Autodesk Inventor part; units mm, degrees
ref_plane "YZ Plane" through (0, 0, 0) normal (1, 0, 0) x (0, 1, 0)
ref_plane "XZ Plane" through (0, 0, 0) normal (0, 1, 0) x (-1, 0, 0)
ref_plane "XY Plane" through (0, 0, 0) normal (0, 0, 1) x (1, 0, 0)
sketch "Sketch1" plane through (0, 0, 0) normal (0, 1, 0) x (-1, 0, 0)
  line L0 (0, 0) -> (20, 0)
  line L1 (20, 0) -> (20, -20)
  line L2 (20, -20) -> (0, -20)
  line L3 (0, -20) -> (0, 0)
  dimension "d0" = 20
  dimension "d1" = 20
extrude "Extrusion1" add sketch "Sketch1" along normal blind 2
sketch "Sketch2" plane through (0, 2, 0) normal (0, 1, 0) x (1, 0, 0)
  line L0 (0, 20) -> (-20, 20)
  line L1 (-20, 20) -> (-20, 0)
  line L2 (-20, 0) -> (0, 0)
  line L3 (0, 0) -> (0, 20)
  line L4 (-18, 2) -> (-18, 18)
  line L5 (-18, 18) -> (-2, 18)
  line L6 (-2, 18) -> (-2, 2)
  line L7 (-2, 2) -> (-18, 2)
  line L8 (-16.75, 16.75) -> (-16.75, 3.25)
  line L9 (-16.75, 3.25) -> (-3.25, 3.25)
  line L10 (-3.25, 3.25) -> (-3.25, 16.75)
  line L11 (-3.25, 16.75) -> (-16.75, 16.75)
  dimension "d4" = 2
  dimension "d5" = 1.25
extrude "Extrusion2" add sketch "Sketch2" along normal blind 2 contours L4 L5 L6 L7
extrude "Extrusion3" cut sketch "Sketch2" against normal blind 10 contours L11 L10 L9 L8
sketch "Sketch3" plane through (0, 0, 0) normal (0, -1, 0) x (1, 0, 0)
  line L0 (-3.25, -3.25) -> (-3.25, -16.75)
  line L1 (-3.25, -16.75) -> (-16.75, -16.75)
  line L2 (-16.75, -16.75) -> (-16.75, -3.25)
  line L3 (-16.75, -3.25) -> (-3.25, -3.25)
  line L4 (0, -20) -> (-20, -20)
  line L5 (0, 0) -> (0, -20)
  line L6 (-20, 0) -> (0, 0)
  line L7 (-20, -20) -> (-20, 0)
  line L8 (-6, -6) -> (-6, -14)
  line L9 (-6, -14) -> (-14, -14)
  line L10 (-14, -14) -> (-14, -6)
  line L11 (-14, -6) -> (-6, -6)
extrude "Extrusion4" add sketch "Sketch3" against normal up to surface (2 mm away) contours L0 L1 L2 L3
extrude "Extrusion5" add sketch "Sketch3" against normal blind 11.5 contours L8 L9 L10 L11
properties part number "latticeChamberCapv4"
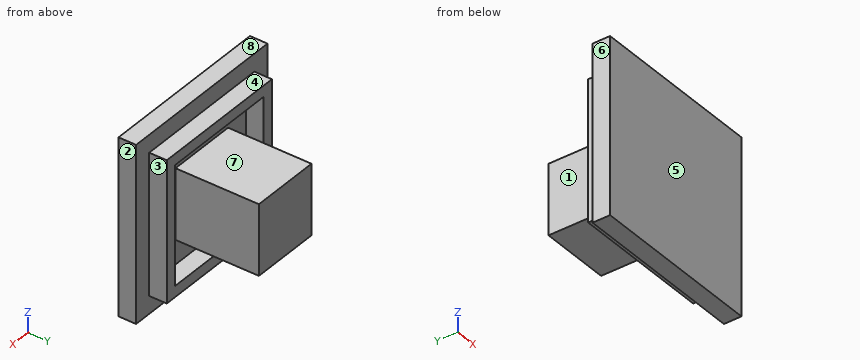
The listing builds one solid part. Answer for the finished solid, in the listing's coordinates (mm). Face numbers are marked on the shaded views. A direction names the side the tool comes from. Coordinates: 2 decimals unless noted, no trailing zeros. Write each loop counter-clockwise with the first axis right and the second up, starting at its lowest first coordinate (ties: lowest second). Pieces come first, ordered by that corner, then holes. Notation, with made-up numbers: (53, 69.5) - (90, 69.5) arc R23 ccw to (90, 98.5) - close; hole circle Ø1 at (29.5, -17.75). An arc over 180 degrees is marked (long way). One line per item, written item: value.
1) A tool of negligible diameter and unlimited length cuts with its end or side. For the marked faces 1, 2, 3, 4 and 5, from which of +Z, -Z, +X, -X, +Y, -Y can it reach the whole face along a straight path? Write none if from no direction.
Geometry check:
face 1: +Y
face 2: +Z, -Z, +X, +Y, -Y
face 3: +Z, -Z, +X, +Y
face 4: +Z, +X, -X, +Y
face 5: +Z, -Z, +X, -X, -Y
2) Find section C-C (y = 7.25). Give the vertices of the cut face in (x, z).
Geometry check:
outline: (-14, -14) - (-6, -14) - (-6, -6) - (-14, -6) - close
3) Each of these flat-tipped pins is pushed along its axis until it touches: pin 1 Ø2 at (y, z) = (3.5, -11.5) entering from -X; pin 2 Ø1.6 at (x, y) = (-7.5, 3.5) entering from +Z; pin 3 Ø3 at (x, z) = (-2.5, -7) entering from +Y. Where does it stop, or does it pass through?
Geometry check:
pin 1: stops at x = -18
pin 2: stops at z = -2
pin 3: stops at y = 4
4) Consider line 1 along X through (y, z) = (3, -12.5); line 2 along X through (y, z) = (2.25, -15). Determine where each line is inside the solid, lowest interval first. Write a range as from..to.
Geometry check:
line 1: x = -18..-16.75, -14..-6, -3.25..-2
line 2: x = -18..-16.75, -3.25..-2
5) Find section B-B (x = -9.25). Give the vertices of the cut face in (y, z), and give its area (3 significant figures).
Geometry check:
outline: (0, -20) - (2, -20) - (2, -18) - (4, -18) - (4, -16.75) - (2, -16.75) - (2, -14) - (11.5, -14) - (11.5, -6) - (2, -6) - (2, -3.25) - (4, -3.25) - (4, -2) - (2, -2) - (2, 0) - (0, 0) - close
area: 121 mm2
6) Find section D-D (x = -17). Give the vertices of the cut face in (y, z), and give its area (3 significant figures).
Geometry check:
outline: (0, -20) - (2, -20) - (2, -18) - (4, -18) - (4, -2) - (2, -2) - (2, 0) - (0, 0) - close
area: 72.0 mm2
7) For a pull along Z with two mould halves and no side action, classify the marked faces 6, 7 and 8 as pulls with the +Z half, pulls with the -Z half, needs draft (parallel to the pull), parting line crosses it, or undercut.
Geometry check:
face 6: needs draft
face 7: undercut
face 8: pulls with the +Z half
8) Find section A-A (z = -15.75). Give the vertices of the cut face in (x, y).
Geometry check:
outline: (-20, 0) - (0, 0) - (0, 2) - (-2, 2) - (-2, 4) - (-3.25, 4) - (-3.25, 2) - (-16.75, 2) - (-16.75, 4) - (-18, 4) - (-18, 2) - (-20, 2) - close
